CAD build for the part. Positions are in the model's coordinates, mm. Give positions to 0.01 mm unless a question says otherwise; leave off trailing zeros. Loops run counter-clockwise (first coordinate to the right, second up) from the corner with the lowest first, then second, coordinate; pieces in that order, holes last. Notation, with made-up numbers: M 2.25,-29 L 59.25,-29 A23 ccw 59.25,2 Z; hole C -18.5,28.25 d9. An arc over 180 degrees is marked long. Answer as CSV lines item,"result".
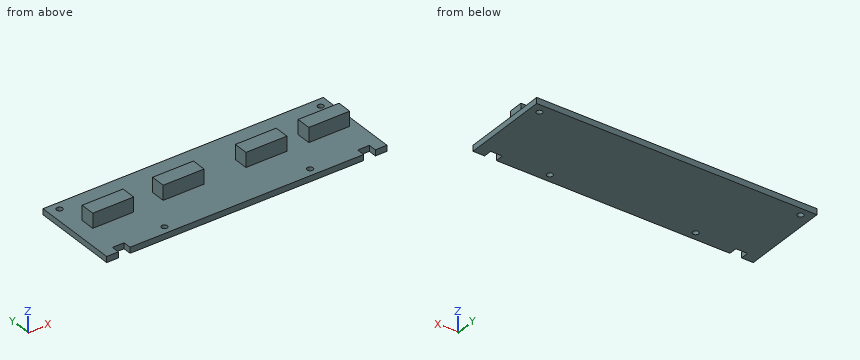
from build123d import *

# Parameters (mm, degrees)
F1_DEPTH = 2
F2_W     = 14
F2_H     = 5
F3_DEPTH = 5
F4_R     = 1
F5_DEPTH = 25


with BuildPart() as f1:
    # F0 (on Top) → F1 (new body)
    with BuildSketch(Plane.XY):
        Polygon((43.908193, 16.15281), (-52.091807, 16.15281), (-52.091807, -13.84719), (-48.091807, -13.84719), (-48.091807, -11.021232), (-44.091807, -11.021232), (-44.091807, -13.84719), (35.908193, -13.84719), (35.908193, -11.021232), (39.908193, -11.021232), (39.908193, -13.84719), (43.908193, -13.84719), align=None)
    extrude(amount=F1_DEPTH)

    # F2 (on face) → F3 (join)
    with BuildSketch(Plane.XY.offset(2)):
        with Locations((-39.782549, 2.5)):
            Rectangle(F2_W, F2_H)
        with Locations((-15.670858, 2.5)):
            Rectangle(F2_W, F2_H)
        with Locations((12.684493, 2.5)):
            Rectangle(F2_W, F2_H)
        with Locations((34.192123, 2.5)):
            Rectangle(F2_W, F2_H)
    extrude(amount=F3_DEPTH)

    # F4 (on face) → F5 (cut)
    with BuildSketch(Plane.XY.offset(2)):
        with Locations((-48.480082, 13.330769)):
            Circle(F4_R)
        with Locations((40.715411, 12.995487)):
            Circle(F4_R)
        with Locations((19.645516, -11.021232)):
            Circle(F4_R)
        with Locations((-30.286502, -11.021232)):
            Circle(F4_R)
    extrude(amount=-F5_DEPTH, mode=Mode.SUBTRACT)


solid = f1.part
1) Drill centre lines: line 1 (X direction, y = 1, z = 2.25); line 2 (X direction, y = 12.5, z = 0.5); line 3 (Y direction, x = -9, z = 6). Where is each one in solid material? Low to high. Write a range as from..to.
Answer below:
line 1,"x = -46.78..-32.78, -22.67..-8.67, 5.68..19.68, 27.19..41.19"
line 2,"x = -52.09..-49.04, -47.92..39.85, 41.58..43.91"
line 3,"y = 0..5"
2) Band-saw the part on D-D on x = 25.5. Give the cut face in (y, z), and give its area (3 significant figures).
Answer below:
outline,"M -13.85,0 L 16.15,0 L 16.15,2 L -13.85,2 Z"
area,"60.0 mm^2"
3) Band-saw the part on C-C on y = 9. Give the cut face in (x, z), and give its area (3 significant figures).
Answer below:
outline,"M -52.09,0 L 43.91,0 L 43.91,2 L -52.09,2 Z"
area,"192 mm^2"
4) Band-saw the part on B-B on x = -37. Give the cut face in (y, z), and give its area (3 significant figures).
Answer below:
outline,"M -13.85,0 L 16.15,0 L 16.15,2 L 5,2 L 5,7 L 0,7 L 0,2 L -13.85,2 Z"
area,"85.0 mm^2"
5) Flat gauge pins, fed straight in: pin 1 (1 mm diameter, centred on x = 38, z = 1.5, fed in from -Y); pin 2 (4 mm diameter, centred on x = -1.5, y = 13, fed in from +Z); pin 3 (2.5 mm diameter, centred on x = 34.5, z = 4, fed in from +Y). Where does each tip first touch, or does it go through?
Answer below:
pin 1,"stops at y = -11.02"
pin 2,"stops at z = 2"
pin 3,"stops at y = 5"
6) Band-saw the part on A-A on z = 5.25. Give the cut face in (x, y), and give its area (3 significant figures).
Answer below:
outline,"M -46.78,0 L -32.78,0 L -32.78,5 L -46.78,5 Z; M -22.67,0 L -8.67,0 L -8.67,5 L -22.67,5 Z; M 5.68,0 L 19.68,0 L 19.68,5 L 5.68,5 Z; M 27.19,0 L 41.19,0 L 41.19,5 L 27.19,5 Z"
area,"280 mm^2"
